Model file for the job. Use its own axes, mm. Face numbers are marked on the shaded views. A direction names the side the tool comes from. Give positions to 0.01 mm unless a question says otherwise; leave off trailing zeros. Answer as a JSON object with one key per item and string values. Group by question number.
```python
from build123d import *

# Parameters (mm, degrees)
F0_W     = 15
F0_H     = 15
F1_DEPTH = 55
F4_D     = 9
F4_DEPTH = 8.8
F4_TIP   = 2.7038727856
F5_D     = 9
F5_DEPTH = 8.8
F5_TIP   = 2.7038727856


with BuildPart() as f1:
    # F0 (on Top) → F1 (new body)
    with BuildSketch(Plane.XY):
        with Locations((0, 0.4354127725)):
            Rectangle(F0_W, F0_H)
    extrude(amount=F1_DEPTH)

    # F4
    with Locations(Plane(origin=(0, 0, 0), x_dir=(1, 0, 0), z_dir=(0, 0, -1))):
        with Locations((0, 0)):
            Hole(F4_D / 2, depth=F4_DEPTH)
            with Locations((0, 0, -(F4_DEPTH + F4_TIP / 2))):  # 118° drill point
                Cone(0, F4_D / 2, F4_TIP, mode=Mode.SUBTRACT)

    # F5
    with Locations(Plane.XY.offset(55)):
        with Locations((0, 0)):
            Hole(F5_D / 2, depth=F5_DEPTH)
            with Locations((0, 0, -(F5_DEPTH + F5_TIP / 2))):  # 118° drill point
                Cone(0, F5_D / 2, F5_TIP, mode=Mode.SUBTRACT)


solid = f1.part
```
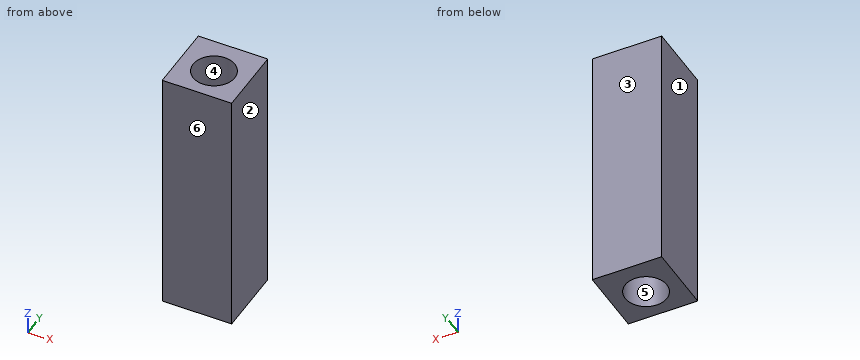
Q1. Wall check: L1, parallel to X at y = 0, z = 52.75; L2, parallel to Y at x = 0, z = 4.25; L3, parallel to X at y = 2.5, z = 52. Give the ranges that are in metal, low to high.
Q2. 3-axis set-ups, long thin cutter, end or side, ignore diameter. For the marked faces 5 and 6: which of +Z, -Z, +X, -X, +Y, -Y reach the whole face in a straight line?
Q3. Drop flat-ended pins along their axis: P1, Ø1, axis at x = 5, y = 0.5, coming from the -Z side; P2, Ø5, axis at x = 0, y = -0.5, coming from the +Z side. Give the stop position or say it passes through.
Q4. Two-plate mould, pull along X, no slides. Class the marked faces 1, 2, 3 and 4: +X half, -X half, draft (parallel to the pull), parting line (faces both ways), or undercut.
Solved:
{
 "1": {"L1": "x = -7.5 to -4.5, 4.5 to 7.5", "L2": "y = -7.06 to -4.5, 4.5 to 7.94", "L3": "x = -7.5 to -3.74, 3.74 to 7.5"},
 "2": {"face 5": "-Z", "face 6": "+Z, -Z, +X, -X, -Y"},
 "3": {"P1": "stops at z = 0", "P2": "stops at z = 45.3"},
 "4": {"face 1": "-X half", "face 2": "+X half", "face 3": "draft", "face 4": "undercut"}
}
